from build123d import *

# Parameters (mm, degrees)
SKETCH_1_W      = 81
SKETCH_1_H      = 81
EXTRUDE_1_DEPTH = 8
FILLET_1_R      = 20
FILLET_2_R      = 10


with BuildPart() as part:
    # 草图1 → 凸台-拉伸1 (new, symmetric)
    with BuildSketch(Plane.XY):
        Polygon((-70, 0), (70, 0), (70, 75), (140, 75), (140, 130), (120, 130), (120, 137), (100, 137), (100, 130), (-100, 130), (-100, 137), (-120, 137), (-120, 130), (-140, 130), (-140, 75), (-70, 75), align=None)
        with Locations((0, 54.5)):
            Rectangle(SKETCH_1_W, SKETCH_1_H, mode=Mode.SUBTRACT)
    extrude(amount=EXTRUDE_1_DEPTH, both=True)

    # 圆角1
    fillet_1_edges = [part.edges().sort_by_distance(p)[0] for p in [
        (70, 0, 0),
        (-70, 0, 0),
        (-70, 75, 0),
        (-140, 75, 0),
        (140, 75, 0),
        (70, 75, 0),
    ]]
    fillet(fillet_1_edges, radius=FILLET_1_R)

    # 圆角2
    fillet_2_edges = [part.edges().sort_by_distance(p)[0] for p in [
        (-40.5, 95, 0),
        (-40.5, 14, 0),
        (40.5, 14, 0),
        (40.5, 95, 0),
    ]]
    fillet(fillet_2_edges, radius=FILLET_2_R)


solid = part.part
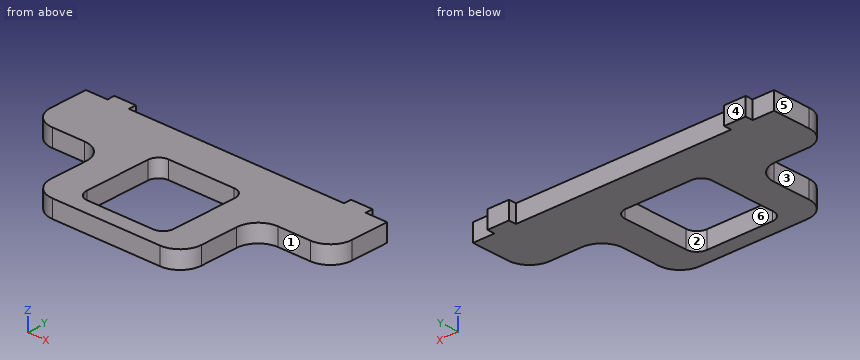
Here's how the part is built. I have some questions about the finished solid (model axes, mm). Face numbers are marked on the shaded views. A direction names the side the tool comes from. Coordinates: 2 decimals unless noted, no trailing zeros. Order: outer loops, then holes, each group sorted by start corner. A loop starts at its lowest first (then second) coordinate and runs counter-clockwise, first axis right, second up.
Item 1: If we mould it in two halves opening along X, with no side actions, what happens to the marked faces 4, 5 and 6? For each: +X half, -X half, draft (parallel to the pull), parting line (faces both ways), or undercut.
Result sheet:
face 4: draft
face 5: -X half
face 6: undercut
Item 2: If we section it at D-D on x = 107: List the corners of the cut face in (y, z) for me.
Result sheet:
outline: (75, -8) - (137, -8) - (137, 8) - (75, 8) - close
Item 3: For the marked faces 1, 2 and 3, which set-ups out of +Z, -Z, +X, -X, +Y, -Y let a thin tool reach every point of the face, with its end or its side?
Result sheet:
face 1: +Z, -Z, +X, -Y
face 2: +Z, -Z
face 3: +Z, -Z, -X, -Y
Item 4: If we section it at A-A on y = 79: List the corners of the cut face in (x, z) for me, plus the area to 3 significant figures.
Result sheet:
outline: (-132, -8) - (-40.5, -8) - (-40.5, 8) - (-132, 8) - close; (40.5, -8) - (132, -8) - (132, 8) - (40.5, 8) - close
area: 2,930 mm2
Item 5: For P1, Ø3.5, axis at y = 134, z = -2, coming from the -X side; P2, Ø5, axis at y = 27.5, z = -1.5, coming from the -X side; P3, Ø5.5, axis at y = 133, z = -2, coming from the +X side, each with a flat end and sliding along its axis, tell me the tip position at first contact or that it passes through.
Result sheet:
P1: stops at x = -120
P2: stops at x = -70
P3: stops at x = 120
Item 6: If we section it at B-B on x = 2: List the corners of the cut face in (y, z) for me.
Result sheet:
outline: (0, -8) - (14, -8) - (14, 8) - (0, 8) - close; (95, -8) - (130, -8) - (130, 8) - (95, 8) - close
Item 7: I need wall thicknesses on line 1 (Y direction, x = -20.5, z = 1); line 2 (X direction, y = 33, z = -1.75); line 3 (Y direction, x = -113.5, z = -2.5). Which ranges of each line are inside material? Lowest first, please.
Result sheet:
line 1: y = 0 to 14, 95 to 130
line 2: x = -70 to -40.5, 40.5 to 70
line 3: y = 75 to 137
